Check sheet for the modelled part. Datum: model origin and axes. Units: mm. Face numbers are marked on the shaded views. A direction names the side the tool comes from. Give positions to 0.01 mm unless a question says otherwise; leave off trailing zeros. Write each loop counter-clockwise with the first axis right and the second up, starting at its lowest first coordinate (ties: lowest second). Pieces come first, ordered by that corner, then holes. Notation, with made-up numbers: (11, 75.5) - (25, 75.5) arc R28 ccw to (25, 97.5) - close; hole circle Ø10 at (88, 58.25). An arc over 180 degrees is marked (long way). Return JSON: item names as keys, results as strings. Group by question number.
```python
from build123d import *

# Parameters (mm, degrees)
SKETCH1_W           = 160
SKETCH1_H           = 80
BOSS_EXTRUDE1_DEPTH = 15
SKETCH2_R           = 7.550070769
SKETCH2_R_2         = 7.255415261
BOSS_EXTRUDE2_DEPTH = 15


with BuildPart() as part:
    # Sketch1 → Boss-Extrude1 (new body)
    with BuildSketch(Plane.XY):
        with Locations((80, 40)):
            Rectangle(SKETCH1_W, SKETCH1_H)
    extrude(amount=BOSS_EXTRUDE1_DEPTH)

    # Sketch2 → Boss-Extrude2 (add)
    with BuildSketch(Plane(origin=(0, 80, 0), x_dir=(1, 0, 0), z_dir=(0, 1, 0))):
        with BuildLine():
            ThreePointArc((112.765660055, 41.575459997), (133.290805297, 17.274846503), (160, 0))
            Line((160, 0), (0, 0))
            ThreePointArc((0, 0), (26.372008671, 16.953021182), (45.778792932, 41.575459997))
            Line((45.778792932, 41.575459997), (112.765660055, 41.575459997))
        make_face()
        with Locations(Location((97.257304614, 22.969928459, 0), (0, 0, 270))):
            Circle(SKETCH2_R, mode=Mode.SUBTRACT)
        with Locations(Location((54.653333848, 22.969928459, 0), (0, 0, 270))):
            Circle(SKETCH2_R_2, mode=Mode.SUBTRACT)
    extrude(amount=-BOSS_EXTRUDE2_DEPTH)


solid = part.part
```
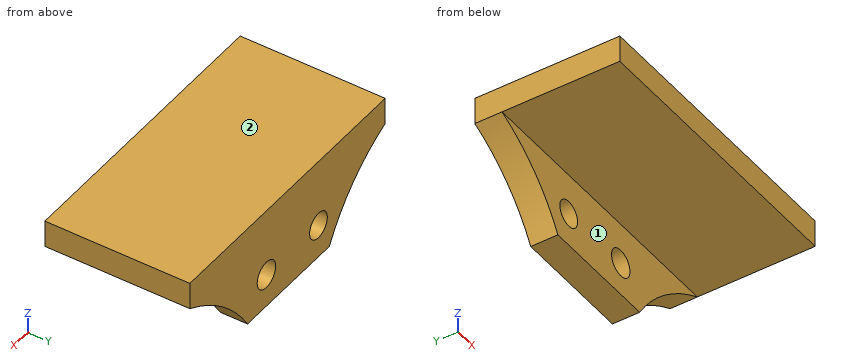
Item 1: Depth check by flat-ended pin: pin 1 (10 mm diameter, centred on x = 20, z = -2.5, fed in from -Y); pin 2 (4 mm diameter, centred on x = 97, y = 25.5, fed in from -Z); pin 3 (6 mm diameter, centred on y = 62.5, z = -23.5, fed in from -X); pin 4 (4 mm diameter, centred on x = 73, z = -6, fed in from -Y). Enter the tip coordinate at first touch or a pass-through.
Item 2: Material ranges on line 1 along X through (y, z) = (74, -17.5); line 2 along Z through (x, y) = (72, 18); line 3 along Y through (x, z) = (21.5, -7), recorded low to high. Write a range as from..to.
Item 3: Section check A-A on y = 70.5. Record the cut outline in (x, z).
Item 4: Section check D-D on y = 62.5. Record the cut outline in (x, z).
Item 5: Section check B-B on z = -24.5. Record the cut outline in (x, y).
Item 6: Access from +Z, -Z, +X, -X, +Y, -Y to the whole of each face (thin tool, end or side, straight path). Record for the marked faces 1 and 2.
Item 7: Section check C-C on x = 141.5. Record the cut outline in (y, z), plus the area to 3 significant figures.
Reply:
{
 "1": {"pin 1": "y = 0", "pin 2": "z = 0", "pin 3": "x = 31.37", "pin 4": "y = 65"},
 "2": {"line 1": "26.97..49.89, 59.42..92.05, 102.46..133.04", "line 2": "0..15", "line 3": "65..80"},
 "3": {"outline": "(0, 0) arc R94.87 cw to (45.78, -41.58) - (112.77, -41.58) arc R108.1 cw to (160, 0) - (160, 15) - (0, 15) - close; hole circle Ø14.51 at (54.65, -22.97); hole circle Ø15.1 at (97.26, -22.97)"},
 "4": {"outline": "(0, 0) - (160, 0) - (160, 15) - (0, 15) - close"},
 "5": {"outline": "(33.8, 65) - (47.56, 65) - (47.56, 80) - (33.8, 80) - close; (61.75, 65) - (89.86, 65) - (89.86, 80) - (61.75, 80) - close; (104.65, 65) - (125.84, 65) - (125.84, 80) - (104.65, 80) - close"},
 "6": {"face 1": "-Z, +X, -X, -Y", "face 2": "+Z, +X, -X, +Y, -Y"},
 "7": {"outline": "(0, 0) - (65, 0) - (65, -10.73) - (80, -10.73) - (80, 15) - (0, 15) - close", "area": "1,360 mm²"}
}
